from build123d import *

# Parameters (mm, degrees)
SKETCH_W     = 285
SKETCH_H     = 130
PAD_DEPTH    = 75
THICKNESS_T  = -3
SKETCH001_W  = 22
SKETCH001_H  = 31
POCKET_DEPTH = 5


with BuildPart() as part:
    # Sketch → Pad (new body, symmetric)
    with BuildSketch(Plane.XY):
        Rectangle(SKETCH_W, SKETCH_H)
    extrude(amount=PAD_DEPTH, both=True)

    # Thickness
    thickness_openings = [part.faces().sort_by_distance(p)[0] for p in [
        (0, 0, -75),
    ]]
    offset(amount=THICKNESS_T, openings=thickness_openings)

    # Sketch001 (on Face5 of Thickness) → Pocket (cut)
    with BuildSketch(Plane.XY.offset(75)):
        with Locations((31, 0)):
            Rectangle(SKETCH001_W, SKETCH001_H)
        with Locations((-31, 0)):
            Rectangle(SKETCH001_W, SKETCH001_H)
    extrude(amount=-POCKET_DEPTH, mode=Mode.SUBTRACT)


solid = part.part
Can you work these out from the model? Positions are in its coordinate system, mm. A direction names the side the tool comes from. Give positions to 0.01 mm unless a question says otherwise; leave off trailing zeros. Order: outer loops, then holes, each group sorted by start corner. A loop starts at its lowest first (then second) coordinate and runs counter-clockwise, first axis right, second up. Notation, with made-up numbers: M -20.5,68.25 L 8.5,68.25 A16 ccw 8.5,83.25 Z; hole C 78.25,56.5 d11. An arc over 180 degrees is marked long. Use one line per item in the form item = value.
Item 1: If I drill on line 1 along X through (y, z) = (-58, 28); line 2 along Y through (x, z) = (-125, -62); line 3 along Z through (x, y) = (33.5, 51), over which ranges is the centre line in solid material (lowest first)? Write a range as [from, to].
Values follow:
line_1 = [-142.5, -139.5], [139.5, 142.5]
line_2 = [-65, -62], [62, 65]
line_3 = [72, 75]
Item 2: If we section it at A-A, the plane x = -33.5: Write out the boundary of the cut face in (y, z).
Values follow:
outline = M -65,-75 L -62,-75 L -62,72 L -15.5,72 L -15.5,75 L -65,75 Z; M 15.5,72 L 62,72 L 62,-75 L 65,-75 L 65,75 L 15.5,75 Z
Item 3: Thinking about a two-plate mould opening in X: for faces 1 (the flat face through (-139.5, -1, 0)), 2 (the flat face through (142.5, -1, 1)), 3 (the flat face through (-2, 65, 1)), which applies, pulls with the +X half, pulls with the -X half, needs draft (parallel to the pull), parting line crosses it, or undercut?
Values follow:
face_1 = undercut
face_2 = pulls with the +X half
face_3 = needs draft
Item 4: If we section it at D-D, the plane x = -116: Write out the boundary of the cut face in (y, z), and give its area (3 significant figures).
Values follow:
outline = M -65,-75 L -62,-75 L -62,72 L 62,72 L 62,-75 L 65,-75 L 65,75 L -65,75 Z
area = 1,270 mm^2
Item 5: If we section it at B-B, the plane y = 4: Write out the boundary of the cut face in (x, z), and give its area (4 significant figures).
Values follow:
outline = M -142.5,-75 L -139.5,-75 L -139.5,72 L -42,72 L -42,75 L -142.5,75 Z; M -20,72 L 20,72 L 20,75 L -20,75 Z; M 42,72 L 139.5,72 L 139.5,-75 L 142.5,-75 L 142.5,75 L 42,75 Z
area = 1,605 mm^2
Item 6: If we section it at C-C, the plane z = 54.5: Write out the boundary of the cut face in (x, y), and give its area (3 significant figures).
Values follow:
outline = M -142.5,-65 L 142.5,-65 L 142.5,65 L -142.5,65 Z; hole M -139.5,-62 L 139.5,-62 L 139.5,62 L -139.5,62 Z
area = 2,450 mm^2
Item 7: Will this pin go through, and if not, where does the flat tip stop? pin 1 Ø6 at (x, y) = (15.5, -9) entering from -Z.
Values follow:
pin_1 = 72
Item 8: For faces 4 (the flat face through (-2, 1, 75)), 5 (the flat face through (139.5, -1, 0)), which set-ups out of +Z, -Z, +X, -X, +Y, -Y let a thin tool reach every point of the face, with its end or its side?
Values follow:
face_4 = +Z, +X, -X, +Y, -Y
face_5 = -Z
